The figure shows three views and two pictorial views of one solid part (mm, origin at its lowest corner). Answer the questions. Coordinates: 2 decimals unless noted, no trailing zeros. Order: outer loops, then holes, each group sorted by start corner. A loop starts at its lowest first (then second) coordinate and runs counter-clockwise, first axis right, second up. Notation, with made-up numbers: (7.25, 86) -> (26.25, 86) arc R18 cw to (26.25, 90) -> close; hole circle Ø5 at (-17.5, 87.5). An arc over 180 degrees is marked (long way). Return JSON: item names as keys, results as strings. Group by question number.
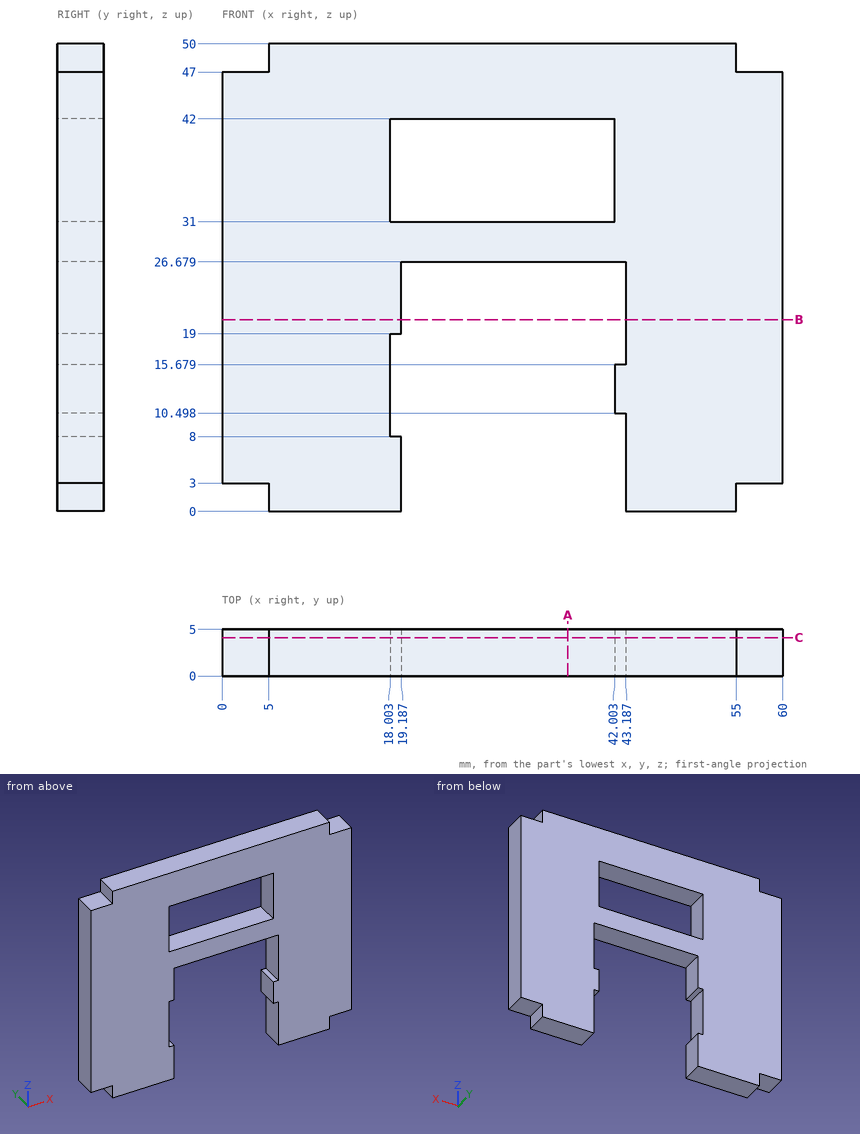
1. Find section C-C on y = 4.1. Determine the outline of the cut face in (x, z).
2. Straight lines are drawn through the part: L1, parallel to Z at x = 36, y = 3.3; L2, parallel to X at y = 0.8, z = 21; L3, parallel to X at y = 4.5, z = 34.5. For each, find the intervals that lie inside material, in ascending order.
3. Find section B-B on z = 20.5. Determine the outline of the cut face in (x, y).
4. Given pin 1 (1.5 mm diameter, centred on y = 1.5, z = 48, fed in from +X); pin 2 (2.5 mm diameter, centred on x = 36, y = 3, fed in from -Z), each flat-ended and moving along its own axis, determine where each tip first touches the part or whether it passes through.
5. Find section A-A on x = 37. Determine the outline of the cut face in (y, z), and give its area (3 significant figures).
Result:
{
 "1": {"outline": "(0, 3) -> (5, 3) -> (5, 0) -> (19.19, 0) -> (19.19, 8) -> (18, 8) -> (18, 19) -> (19.19, 19) -> (19.19, 26.68) -> (43.19, 26.68) -> (43.19, 15.68) -> (42, 15.68) -> (42, 10.5) -> (43.19, 10.5) -> (43.19, 0) -> (55, 0) -> (55, 3) -> (60, 3) -> (60, 47) -> (55, 47) -> (55, 50) -> (5, 50) -> (5, 47) -> (0, 47) -> close; hole (18, 31) -> (42, 31) -> (42, 42) -> (18, 42) -> close"},
 "2": {"L1": "26.68 to 31, 42 to 50", "L2": "0 to 19.19, 43.19 to 60", "L3": "0 to 18, 42 to 60"},
 "3": {"outline": "(0, 0) -> (19.19, 0) -> (19.19, 5) -> (0, 5) -> close; (43.19, 0) -> (60, 0) -> (60, 5) -> (43.19, 5) -> close"},
 "4": {"pin 1": "x = 55", "pin 2": "z = 26.68"},
 "5": {"outline": "(0, 26.68) -> (5, 26.68) -> (5, 31) -> (0, 31) -> close; (0, 42) -> (5, 42) -> (5, 50) -> (0, 50) -> close", "area": "61.6 mm^2"}
}
